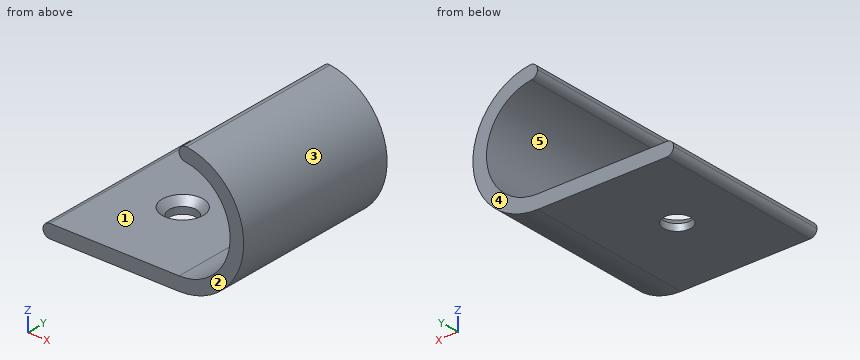
from build123d import *

# Parameters (mm, degrees)
F1_DEPTH = 12.5
F2_R     = 2
F3_DEPTH = 25
F4_SIZE  = 1
F5_R     = 0.99999


# Not quite as in the source:
# - a fillet or chamfer is up to 0.001 mm smaller than in the source, because OpenCascade refuses the exact size


with BuildPart() as f1:
    # F0 (on Front) → F1 (new body, symmetric)
    with BuildSketch(Plane.XZ):
        with BuildLine():
            ThreePointArc((10, 16), (17.5, 8.5), (10, 1))
            Line((10, 1), (-10, 1))
            Line((-10, 1), (-10, -1))
            Line((-10, -1), (10, -1))
            ThreePointArc((10, -1), (19.5, 8.5), (10, 18))
            Line((10, 18), (10, 16))
        make_face()
    extrude(amount=F1_DEPTH, both=True)

    # F2 (on face) → F3 (cut)
    with BuildSketch(Plane(origin=(0, 0, -1), x_dir=(1, 0, 0), z_dir=(0, 0, -1))):
        Circle(F2_R)
    extrude(amount=-F3_DEPTH, mode=Mode.SUBTRACT)

    # F4
    f4_edges = [f1.edges().sort_by_distance(p)[0] for p in [
        (-2, 0, 1),
    ]]
    chamfer(f4_edges, length=F4_SIZE)

    # F5 (radius 1 in the source; OpenCascade refuses exactly that, so slightly less here)
    f5_edges = [f1.edges().sort_by_distance(p)[0] for p in [
        (10, 0, 18),
        (10, 0, 16),
        (-10, 0, 1),
        (-10, 0, -1),
    ]]
    fillet(f5_edges, radius=F5_R)


solid = f1.part
Source: CAD feature listing. Evaluate the final solid. Frame: model axes, mm. Face numbers are marked on the shaded views. A direction names the side the tool comes from. Round coordinates to 2 decimals unless told otherwise and drop trailing zeros. Loops run counter-clockwise (first coordinate to the right, second up) from the corner with the lowest first, then second, coordinate; pieces in that order, holes last. Notation, with made-up numbers: M 78,16.25 L 114,16.25 A28 ccw 114,48.25 Z; hole C -14,81.25 d5. An arc over 180 degrees is marked long. Return JSON: item names as keys, results as strings. Group by question number.
1. Material intervals for line 1 along Y through (x, z) = (0, -0.5); line 2 along Z through (x, y) = (13.5, -8.25); line 3 along Z through (x, y) = (-5.5, -1.25), sorted ascending. Write a range as from..to.
2. Mould query, pull axis Z, two halves, no side actions, for the marked faces 3, 4 and 5. Classes: released by +Z, released by -Z, zero draft, split by the parting line, or undercut.
3. Section query B-B on x = 0. Output: boundary loops of the cut face in (y, z).
4. Pin query (flat end, axial travel): pin 1 (3 mm diameter, centred on y = -3, z = 13, fed in from -X); pin 2 (8 mm diameter, centred on x = -2, y = 5, fed in from +Z); pin 3 (2 mm diameter, centred on x = 16, y = 1, fed in from -Z). Return the tip coordinate at first contact, or that it passes through.
5. Section query D-D on z = 8.5. Output: boundary loops of the cut face in (x, y).
6. Reachability of the marked faces 1 and 2 from +Z, -Z, +X, -X, +Y, -Y: full face, straight path, thin tool, end or side. Return the list, or none.
Checks:
{
 "1": {"line 1": "y = -12.5..-2, 2..12.5", "line 2": "z = -0.33..1.87, 15.13..17.33", "line 3": "z = -1..1"},
 "2": {"face 3": "split by the parting line", "face 4": "zero draft", "face 5": "undercut"},
 "3": {"outline": "M -12.5,-1 L -2,-1 L -2,0 L -3,1 L -12.5,1 Z; M 2,-1 L 12.5,-1 L 12.5,1 L 3,1 L 2,0 Z"},
 "4": {"pin 1": "stops at x = 14.5", "pin 2": "stops at z = 1", "pin 3": "stops at z = 0.42"},
 "5": {"outline": "M 17.5,-12.5 L 19.5,-12.5 L 19.5,12.5 L 17.5,12.5 Z"},
 "6": {"face 1": "+Z, -X, +Y, -Y", "face 2": "+Z, -Z, +X, -X, -Y"}
}
